Here's how the part is built. I have some questions about the finished solid (model axes, mm). A direction names the side the tool comes from. Give positions to 0.01 mm unless a question says otherwise; leave off trailing zeros. Loops run counter-clockwise (first coordinate to the right, second up) from the corner with the lowest first, then second, coordinate; pieces in that order, holes last. Notation, with made-up numbers: M 62.5,44.5 L 69.5,44.5 A19 cw 69.5,52.5 Z; hole C -32.5,-19.75 d1. An arc over 180 degrees is marked long. Answer as CSV lines item,"result". Start each with the question number.
Item 1: If I drill on line 1 along X through (y, z) = (-25, 47.25) (3 decimals); line 2 along Y through (x, z) = (-50, 43) (3 decimals); line 3 along Y through (x, z) = (50, 44) (3 decimals), over which ranges is the centre line in solid material (lowest first)? Write a range as from..to.
Item 2: I want a section at C-C on y = 33.5. List the corners of the cut face in (x, z) for me.
Item 3: Will these pins go through, and if not, where does the flat tip stop? P1, Ø4, axis at x = 18.5, y = -23, coming from the +Z side; P2, Ø6, axis at x = -43.5, y = -27.5, coming from the -Z side; P3, Ø3, axis at x = -49, y = 25, coming from the +Z side.
Item 4: I want a section at A-A on y = 11.5. List the corners of the cut face in (x, z) for me, plus the area to 3 significant figures.
Item 5: For faces 4 (the cylindrical face through (-44.88, 24.77, 44.97)), 5 (the flat face through (-1, 1, 0)), which set-ups out of +Z, -Z, +X, -X, +Y, -Y let a thin tool reach every point of the face, with its end or its side?
Item 6: I want a section at D-D on x = -50. List the corners of the cut face in (y, z) for me (3 decimals).
Item 7: If we mould it in two halves opening along X, with no side actions, what happens to faces 1 (the flat face through (50, 1, 50)), 2 (the cylindrical face through (-0.77, -32.61, 15.01)), 3 (the flat face through (-60, -1, 25))? For each: released by +X, released by -X, zero draft, split by the parting line, or undercut.
Item 8: I want a section at B-B on x = 0. List the corners of the cut face in (y, z) for me.
from build123d import *

# Parameters (mm, degrees)
SKETCH1_W           = 120
SKETCH1_H           = 80
BOSS_EXTRUDE1_DEPTH = 50
SKETCH3_R           = 5.125
CUT_EXTRUDE1_DEPTH  = 10.2


with BuildPart() as part:
    # Sketch1 → Boss-Extrude1 (new body)
    with BuildSketch(Plane.XY):
        Rectangle(SKETCH1_W, SKETCH1_H)
    extrude(amount=BOSS_EXTRUDE1_DEPTH)

    # Sketch3 → Cut-Extrude1 (cut)
    with BuildSketch(Plane.XY.offset(50)):
        with Locations(Location((-50, 25, 0), (0, 0, 180))):
            Circle(SKETCH3_R)
        with Locations(Location((50, -25, 0), (0, 0, 180))):
            Circle(SKETCH3_R)
    extrude(amount=-CUT_EXTRUDE1_DEPTH, mode=Mode.SUBTRACT)

    # Sketch2 → Cut-Revolve1 (revolve, cut)
    with BuildSketch(Plane.XY.offset(50)):
        with BuildLine():
            Line((-35, 40), (-35, 25))
            Line((-35, 25), (-46.913025467, 5.144957554))
            ThreePointArc((-46.913025467, 5.144957554), (-48.33809621, 0), (-46.913025467, -5.144957554))
            Line((-46.913025467, -5.144957554), (-35, -25))
            Line((-35, -25), (-35, -40))
            Line((-35, -40), (0, -40))
            Line((0, -40), (0, 40))
            Line((0, 40), (-35, 40))
        make_face()
    revolve(axis=Axis((0, 40, 50), (0, -1, 0)), mode=Mode.SUBTRACT)


solid = part.part
Result:
1,line 1,"-60..-34.892, 34.892..44.875, 55.125..60"
1,line 2,"-40..19.875, 30.125..40"
1,line 3,"-40..-30.125, -19.875..40"
2,outline,"M -60,0 L 60,0 L 60,50 L 35,50 A35 cw -35,50 L -60,50 Z"
3,P1,"z = 20.79"
3,P2,"z = 0"
3,P3,"z = 39.8"
4,outline,"M -60,0 L 60,0 L 60,50 L 43.1,50 A43.1 cw -43.1,50 L -60,50 Z"
4,area,"3,080 mm^2"
5,face 4,"+Z"
5,face 5,"-Z, +X, -X, +Y, -Y"
6,outline,"M -40,0 L 40,0 L 40,50 L 30.125,50 L 30.125,39.8 L 19.875,39.8 L 19.875,50 L -40,50 Z"
7,face 1,"zero draft"
7,face 2,"undercut"
7,face 3,"released by -X"
8,outline,"M -40,0 L 40,0 L 40,15 L 25,15 L 5.14,3.09 A10 cw -5.14,3.09 L -25,15 L -40,15 Z"
